from build123d import *

# Parameters (mm, degrees)
F0_W      = 385
F0_H      = 270
F1_DEPTH  = 50
F2_W      = 239.333302365
F2_H      = 175.5943608609
F2_W_2    = 179.333302365
F2_H_2    = 115.5943608609
F3_DEPTH  = 2
F4_R      = 32.5
F5_DEPTH  = 25
F6_W      = 50
F6_H      = 30
F7_DEPTH  = 10
F8_SIZE   = 25
F9_R      = 5
F10_R     = 15
F11_DEPTH = 50
F13_D     = 4.2
F13_DEPTH = 10
F13_TIP   = 1.2618073
F14_R     = 5


with BuildPart() as f1:
    # F0 (on Front) → F1 (new body)
    with BuildSketch(Plane.XZ):
        with Locations((0, 135)):
            Rectangle(F0_W, F0_H)
    extrude(amount=F1_DEPTH)

    # F2 (on face) → F3 (join)
    with BuildSketch(Plane.XZ.offset(50)):
        with Locations((-37.8333488175, 132.7971804305)):
            Rectangle(F2_W, F2_H)
        with Locations((-37.8333488175, 132.7971804305)):
            Rectangle(F2_W_2, F2_H_2, mode=Mode.SUBTRACT)
    extrude(amount=F3_DEPTH)

    # F4 (on face) → F5 (join)
    with BuildSketch(Plane.XZ.offset(50)):
        with Locations((137.5, 195)):
            Circle(F4_R)
    extrude(amount=F5_DEPTH)

    # F6 (on face) → F7 (join)
    with BuildSketch(Plane.XZ.offset(50)):
        with Locations((142.5, 90)):
            Rectangle(F6_W, F6_H)
        with Locations((142.5, 45)):
            Rectangle(F6_W, F6_H)
    extrude(amount=F7_DEPTH)

    # F8
    f8_edges = [f1.edges().sort_by_distance(p)[0] for p in [
        (192.5, -25, 270),
        (-192.5, -25, 270),
        (-192.5, -25, 0),
        (192.5, -25, 0),
    ]]
    chamfer(f8_edges, length=F8_SIZE)

    # F9
    f9_edges = [f1.edges().sort_by_distance(p)[0] for p in [
        (105, -75, 195),
    ]]
    fillet(f9_edges, radius=F9_R)

    # F10 (on face) → F11 (join)
    with BuildSketch(Plane(origin=(0, 0, 0), x_dir=(1, 0, 0), z_dir=(0, 0, -1))):
        with Locations((117.5, 25)):
            Circle(F10_R)
    extrude(amount=F11_DEPTH)

    # F13
    with Locations(Plane(origin=(0, 0, 0), x_dir=(-1, 0, 0), z_dir=(0, 1, 0))):
        with Locations((-37.5, 175), (37.5, 175), (37.5, 100), (-37.5, 100)):
            Hole(F13_D / 2, depth=F13_DEPTH)
            with Locations((0, 0, -(F13_DEPTH + F13_TIP / 2))):  # 118° drill point
                Cone(0, F13_D / 2, F13_TIP, mode=Mode.SUBTRACT)

    # F14
    f14_edges = [f1.edges().sort_by_distance(p)[0] for p in [
        (0, 0, 270),
        (180, 0, 257.5),
        (192.5, 0, 135),
        (180, 0, 12.5),
        (0, 0, 0),
        (-180, 0, 257.5),
        (-192.5, 0, 135),
        (-180, 0, 12.5),
        (180, -50, 257.5),
        (192.5, -50, 135),
        (180, -50, 12.5),
        (0, -50, 0),
        (-180, -50, 12.5),
        (-192.5, -50, 135),
        (-180, -50, 257.5),
        (0, -50, 270),
    ]]
    fillet(f14_edges, radius=F14_R)


solid = f1.part
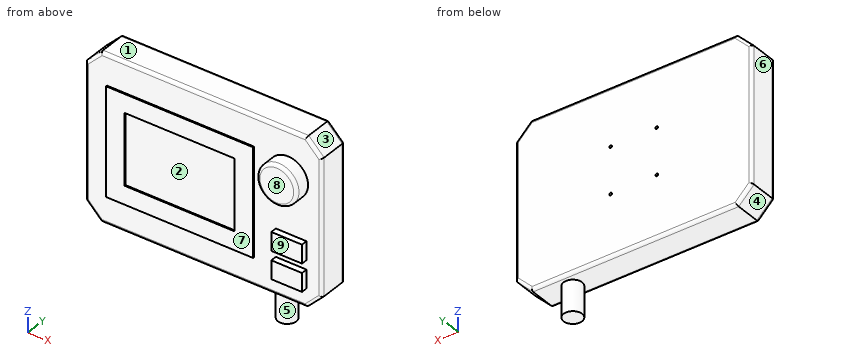
Read the model definition and answer for the solid it produces. Units are mm, in the model's axes. Face numbers are marked on the shaded views. A direction names the side the tool comes from. Round coordinates to 2 decimals unless told otherwise and drop trailing zeros. Write each loop counter-clockwise with the first axis right and the second up, starting at its lowest first coordinate (ties: lowest second). Pieces come first, ordered by that corner, then holes. Notation, with made-up numbers: M -34,86 L 22,86 A24 cw 22,125 Z; hole C -11,69 d3. An arc over 180 degrees is marked long. Use a Markdown table: item, result.
1) For a pull along X with two mould halves and no side action, classify the marked faces 1, 2, 3 and 4 as pulls with the +X half, pulls with the -X half, needs draft (parallel to the pull), parting line crosses it, or undercut.
Answers follow:
| item | result |
|---|---|
| face 1 | needs draft |
| face 2 | undercut |
| face 3 | pulls with the +X half |
| face 4 | pulls with the -X half |
2) The part is cut by section C-C (x = 137.5). Write down the section's boundary in (y, z), plus the area to 3 significant figures.
Answers follow:
| item | result |
|---|---|
| outline | M -75,167.5 A5 ccw -70,162.5 L -50,162.5 L -50,105 L -60,105 L -60,75 L -50,75 L -50,60 L -60,60 L -60,30 L -50,30 L -50,5 A5 ccw -45,0 L -5,0 A5 ccw 0,5 L 0,265 A5 ccw -5,270 L -45,270 A5 ccw -50,265 L -50,227.5 L -70,227.5 A5 ccw -75,222.5 Z |
| area | 15,700 mm2 |
3) A tool of negligible diameter and unlimited length cuts with its end or side. For the marked faces 5, 6, 7, 8 and 9, from which of +Z, -Z, +X, -X, +Y, -Y can it reach the whole face along a straight path? Write none if from no direction.
Answers follow:
| item | result |
|---|---|
| face 5 | -Z |
| face 6 | +Z, -Z, -X, +Y, -Y |
| face 7 | +Z, -Z, -X, -Y |
| face 8 | +Z, -Z, +X, -X, -Y |
| face 9 | -Z, +X, -X, -Y |
4) The part is cut by section D-D (x = 30.5). Write down the section's boundary in (y, z).
Answers follow:
| item | result |
|---|---|
| outline | M -52,45 L -50,45 L -50,5 A5 ccw -45,0 L -5,0 A5 ccw 0,5 L 0,265 A5 ccw -5,270 L -45,270 A5 ccw -50,265 L -50,220.59 L -52,220.59 L -52,190.59 L -50,190.59 L -50,75 L -52,75 Z |
5) The part is cut by section B-B (y = -25). Write down the section's boundary in (x, z), plus the area to 3 significant figures.
Answers follow:
| item | result |
|---|---|
| outline | M -192.5,25 L -167.5,0 L 102.5,0 L 102.5,-50 L 132.5,-50 L 132.5,0 L 167.5,0 L 192.5,25 L 192.5,245 L 167.5,270 L -167.5,270 L -192.5,245 Z |
| area | 104,000 mm2 |
6) Straight lines are drawn through the part: line 1 along Z through (x, y) = (-37, -4); line 2 along X through (y, z) = (-7.25, 175); line 3 along Z through (x, y) = (-37.5, -6.5). For each, find the intervals that lie inside material, in ascending order. Write a range as [from, to].
Answers follow:
| item | result |
|---|---|
| line 1 | z = [0.1, 97.96], [102.04, 172.96], [177.04, 269.9] |
| line 2 | x = [-192.5, -39.6], [-35.4, 35.4], [39.6, 192.5] |
| line 3 | z = [0, 97.9], [102.1, 172.9], [177.1, 270] |
7) The part is cut by section A-A (z = 195). Write down the section's boundary in (x, y), plus the area to 3 significant figures.
Answers follow:
| item | result |
|---|---|
| outline | M -192.5,-45 A5 ccw -187.5,-50 L -157.5,-50 L -157.5,-52 L 81.83,-52 L 81.83,-50 L 105,-50 L 105,-70 A5 ccw 110,-75 L 165,-75 A5 ccw 170,-70 L 170,-50 L 187.5,-50 A5 ccw 192.5,-45 L 192.5,-5 A5 ccw 187.5,0 L -187.5,0 A5 ccw -192.5,-5 Z |
| area | 21,300 mm2 |
8) Flat-ended cylindrical pins translate along their axes: pin 1 (1 mm diameter, centred on x = -51, y = -51, fed in from -Z); pin 2 (6 mm diameter, centred on x = -86.5, z = 5, fed in from -Y); pin 3 (3 mm diameter, centred on x = 139.5, y = -56.5, fed in from +Z); pin 4 (1.5 mm diameter, centred on y = -61.5, z = 86.5, fed in from -X). Find the tip coordinate at first contact, or state that the pin passes through.
Answers follow:
| item | result |
|---|---|
| pin 1 | stops at z = 45 |
| pin 2 | stops at y = -50 |
| pin 3 | stops at z = 227.5 |
| pin 4 | passes through |
